```python
from build123d import *

# Parameters (mm, degrees)
SKETCH1_W                                           = 152.4
SKETCH1_H                                           = 50.8
BOSS_EXTRUDE1_DEPTH                                 = 50.8
F_3_4_16_TAPPED_HOLE1_D                             = 17.4625
F_3_4_16_TAPPED_HOLE1_DEPTH                         = 38.1
F_3_4_16_TAPPED_HOLE1_TIP                           = 5.24626428
CBORE_FOR_0_BINDING_HEAD_MACHINE_SCREW2_D           = 16.002
CBORE_FOR_0_BINDING_HEAD_MACHINE_SCREW2_CBORE_D     = 25.4
CBORE_FOR_0_BINDING_HEAD_MACHINE_SCREW2_CBORE_DEPTH = 16.002
CSK_FOR_0_FLAT_HEAD_MACHINE_SCREW_100_D             = 12.7
CSK_FOR_0_FLAT_HEAD_MACHINE_SCREW_100_CSINK_D       = 25.4
CSK_FOR_0_FLAT_HEAD_MACHINE_SCREW_100_CSINK_ANGLE   = 82


with BuildPart() as part:
    # Sketch1 → Boss-Extrude1 (new body)
    with BuildSketch(Plane(origin=(0, 0, 0), x_dir=(1, 0, 0), z_dir=(0, 1, 0))):
        with Locations((76.2, -25.4)):
            Rectangle(SKETCH1_W, SKETCH1_H)
    extrude(amount=BOSS_EXTRUDE1_DEPTH)

    # 3/4-16 Tapped Hole1
    with Locations(Plane(origin=(0, 50.8, 0), x_dir=(1, 0, 0), z_dir=(0, 1, 0))):
        with Locations((127, -25.4)):
            Hole(F_3_4_16_TAPPED_HOLE1_D / 2, depth=F_3_4_16_TAPPED_HOLE1_DEPTH)
            with Locations((0, 0, -(F_3_4_16_TAPPED_HOLE1_DEPTH + F_3_4_16_TAPPED_HOLE1_TIP / 2))):  # 118° drill point
                Cone(0, F_3_4_16_TAPPED_HOLE1_D / 2, F_3_4_16_TAPPED_HOLE1_TIP, mode=Mode.SUBTRACT)

    # CBORE for #0 Binding Head Machine Screw2 (through all)
    with Locations(Plane(origin=(0, 50.8, 0), x_dir=(1, 0, 0), z_dir=(0, 1, 0))):
        with Locations((25.4, -25.4)):
            CounterBoreHole(CBORE_FOR_0_BINDING_HEAD_MACHINE_SCREW2_D / 2, CBORE_FOR_0_BINDING_HEAD_MACHINE_SCREW2_CBORE_D / 2, CBORE_FOR_0_BINDING_HEAD_MACHINE_SCREW2_CBORE_DEPTH)

    # CSK for #0 Flat Head Machine Screw (100)3 (through all)
    with Locations(Plane(origin=(0, 50.8, 0), x_dir=(1, 0, 0), z_dir=(0, 1, 0))):
        with Locations((76.2, -25.4)):
            CounterSinkHole(CSK_FOR_0_FLAT_HEAD_MACHINE_SCREW_100_D / 2, CSK_FOR_0_FLAT_HEAD_MACHINE_SCREW_100_CSINK_D / 2, counter_sink_angle=CSK_FOR_0_FLAT_HEAD_MACHINE_SCREW_100_CSINK_ANGLE)


solid = part.part
```
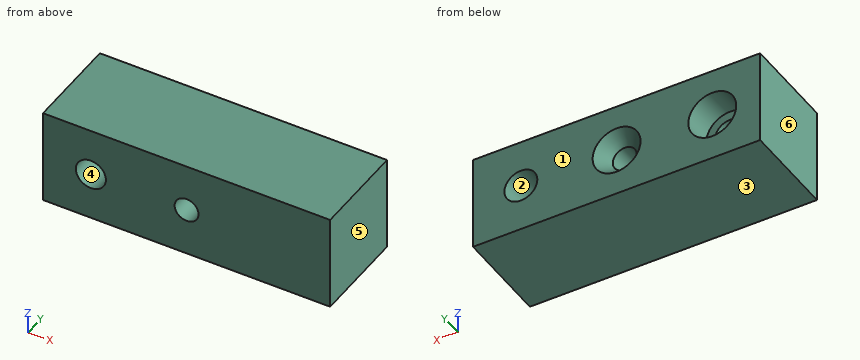
Part model, mm, in its own coordinate system. Face numbers are marked on the shaded views. A direction names the side the tool comes from. Round coordinates to 2 decimals unless told otherwise and drop trailing zeros. Order: outer loops, then holes, each group sorted by start corner. A loop starts at its lowest first (then second) coordinate and runs counter-clockwise, first axis right, second up. Notation, with made-up numbers: M 17,44 L 41,44 A27 cw 41,60 Z; hole C 64,70.25 d3. An arc over 180 degrees is marked long. Answer in a Markdown table with one row per item. Add a question column.
Q1. Wall check: L1, parallel to X at y = 37, z = 25; L2, parallel to X at y = 15, z = 25; L3, parallel to Z at x = 25, y = 13. Give the ranges that are in metal, low to high. Write a range as from..to.
Q2. 3-axis set-ups, long thin cutter, end or side, ignore diameter. For the marked faces 1 and 2: which of +Z, -Z, +X, -X, +Y, -Y reach the whole face in a straight line?
Q3. Cut at B-B on y = 25.5. Give the cut face in (x, z), and give its area (3 significant figures).
Q4. Mould opens along X. For the marked faces 3, 4, 5 and 6 say: +X half, -X half, draft (parallel to the pull), parting line (faces both ways), or undercut.
Q5. Pin check, flat tips, straight feed: pin 1 (22.5 mm diameter, centred on x = 127, z = 25.4, fed in from +Y); pin 2 (7.5 mm diameter, centred on x = 22, z = 22.5, fed in from +Y). Stop position of each tip, or through.
Q6. Cut at D-D on z = 27. Give the number of separate pieces and of enclosed holes in the cut face, and give its area (3 significant figures).
Q7. Cut at C-C on x = 25.4. Give the cut face in (y, z).
Q8. Cut at A-A on x = 76.2. Give the cut face in (y, z), and give its area (3 significant figures).
Established:
| question | item | result |
|---|---|---|
| 1 | L1 | x = 0..12.71, 38.09..69.86, 82.54..118.28, 135.72..152.4 |
| 1 | L2 | x = 0..17.41, 33.39..69.86, 82.54..118.28, 135.72..152.4 |
| 1 | L3 | z = 0..17.41, 33.39..50.8 |
| 2 | face 1 | +Z, -Z, +X, -X, +Y |
| 2 | face 2 | +Y |
| 3 | outline | M 0,0 L 152.4,0 L 152.4,50.8 L 0,50.8 Z; hole C 25.4,25.4 d16; hole C 76.2,25.4 d12.7; hole C 127,25.4 d17.46 |
| 3 | area | 7,170 mm2 |
| 4 | face 3 | draft |
| 4 | face 4 | undercut |
| 4 | face 5 | +X half |
| 4 | face 6 | -X half |
| 5 | pin 1 | stops at y = 50.8 |
| 5 | pin 2 | stops at y = 34.8 |
| 6 | separate pieces | 3 |
| 6 | enclosed holes | 0 |
| 6 | area | 5,430 mm2 |
| 7 | outline | M 0,0 L 50.8,0 L 50.8,12.7 L 34.8,12.7 L 34.8,17.4 L 0,17.4 Z; M 0,33.4 L 34.8,33.4 L 34.8,38.1 L 50.8,38.1 L 50.8,50.8 L 0,50.8 Z |
| 8 | outline | M 0,0 L 50.8,0 L 50.8,12.7 L 43.5,19.05 L 0,19.05 Z; M 0,31.75 L 43.5,31.75 L 50.8,38.1 L 50.8,50.8 L 0,50.8 Z |
| 8 | area | 1,890 mm2 |
